Job drawing, mm, ordinate dimensions from the low corner. One solid piece. A direction names the side the tool comes from. Give positions to 0.01 mm unless a question says otherwise; leave off trailing zeros. Order: outer loops, then holes, each group sorted by start corner. A loop starts at its lowest first (then second) coordinate and runs counter-clockwise, first axis right, second up. Notation, with made-up numbers: M 15.25,34 L 31.25,34 A22 ccw 31.25,48 Z; hole C 22,15 d7. An arc over 180 degrees is marked long. One line per question, with ' | ' between items.
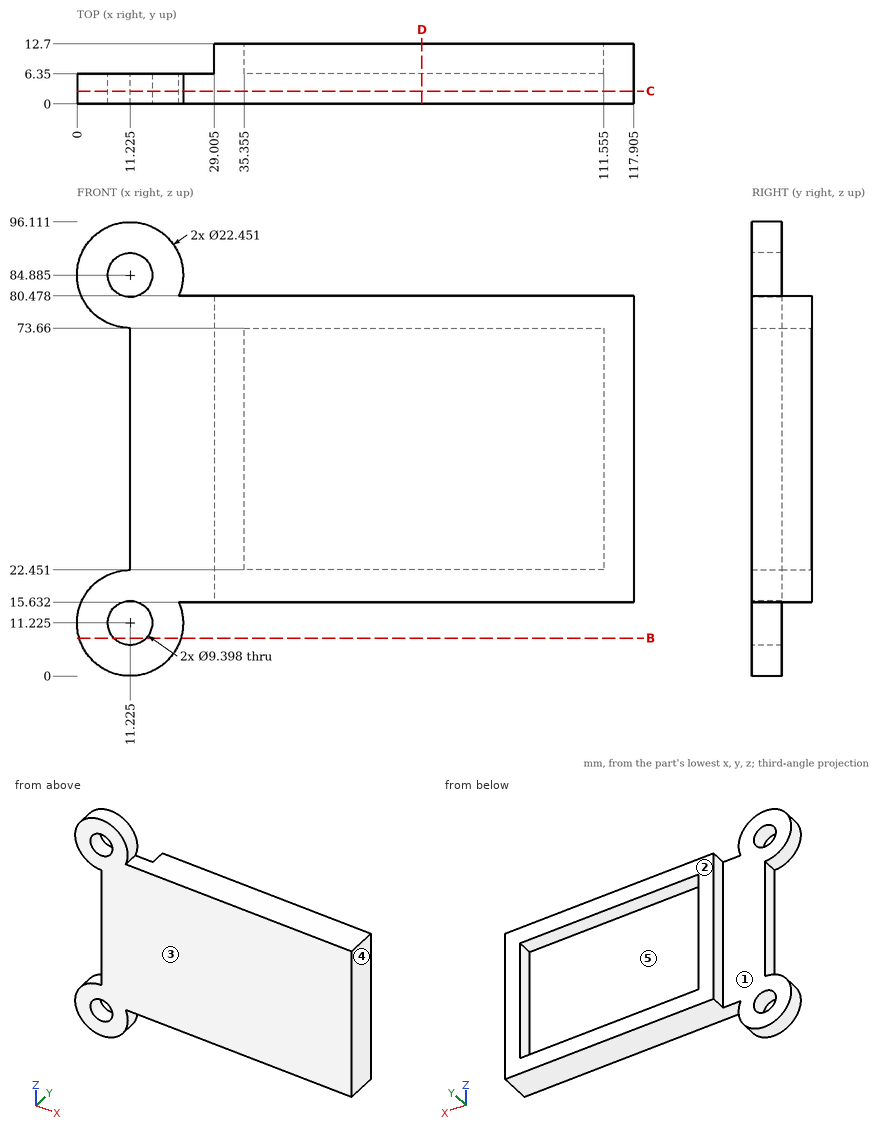
1. Slice it at B-B on z = 8. Give the cut face in (x, y).
Worked out:
outline: M 0.47,0 L 7.81,0 L 7.81,6.35 L 0.47,6.35 Z; M 14.64,0 L 21.98,0 L 21.98,6.35 L 14.64,6.35 Z
2. Slice it at D-D on x = 73. Give the cut face in (y, z).
Worked out:
outline: M 0,15.63 L 12.7,15.63 L 12.7,22.45 L 6.35,22.45 L 6.35,73.66 L 12.7,73.66 L 12.7,80.48 L 0,80.48 Z
3. Probe L1, parallel to Z at x = 106, y = 8.75; L2, parallel to X at y = 10.5, z = 68 (1 decimal); L3, parallel to X at y = 1.25, z = 40.5 (1 decimal). List the from-to ranges inside material, lowest first. Write a range as from..to.
Worked out:
L1: z = 15.63..22.45, 73.66..80.48 | L2: x = 29..35.4, 111.6..117.9 | L3: x = 11.2..117.9
4. Mould opens along X. For the marked faces 3, 4 and 5 say: released by +X, released by -X, zero draft, split by the parting line, or undercut.
Worked out:
face 3: zero draft | face 4: released by +X | face 5: undercut
5. Slice it at C-C on y = 2.75. Give the number of separate pieces and of enclosed holes in the cut face, then the cut area to 3 significant figures.
Worked out:
separate pieces: 1 | enclosed holes: 2 | area: 7,470 mm2
6. Tool access for the marked faces 1 and 2: list every direction of +Z, -Z, +X, -X, +Y, -Y with a clear straight run to the whole face (end or side of a thin tool).
Worked out:
face 1: +Z, -Z, -X, +Y | face 2: +Z, -Z, +X, -X, +Y
7. Drop flat-ended pins along their axis: pin 1 (6.5 mm diameter, centred on x = 87, y = 8.5, fed in from -Z); pin 2 (8.5 mm diameter, centred on x = 11.23, z = 11.23, fed in from -Y); pin 3 (3 mm diameter, centred on y = 8.5, z = 53.5, fed in from -X) (1 decimal); pin 4 (4 mm diameter, centred on x = 85.5, y = 8.5, fed in from +Z). Give the stop position or say it passes through.
Worked out:
pin 1: stops at z = 15.63 | pin 2: passes through | pin 3: stops at x = 29 | pin 4: stops at z = 80.48
